Geometry: final body of the model. Coordinates: model frame, mm. A direction names the side the tool comes from. Coordinates: 2 decimals unless noted, no trailing zeros. Order: outer loops, then holes, each group sorted by start corner. A loop starts at its lowest first (then second) coordinate and runs counter-clockwise, first axis right, second up. Notation, with made-up numbers: (-21, 41) -> (-15, 41) arc R11 ccw to (-15, 45) -> close; hole circle Ø11 at (-16.75, 65.25). An arc over 180 degrees is marked (long way). Use CSV: the item, a comma, the result in double quotes. Start each with the question number.
from build123d import *

# Parameters (mm, degrees)
F0_R          = 35
F1_DEPTH      = 2
F2_R          = 29
F3_DEPTH      = 5
F4_R          = 27
F5_DEPTH      = 5
F6_W          = 45.179169625
F6_H          = 45.1430678368
F7_DEPTH      = 2.001
F7_DEPTH_BACK = 5.001
F8_R          = 4.99999
F9_R          = 10


# Not quite as in the source:
# - a fillet or chamfer is up to 0.001 mm smaller than in the source, because OpenCascade refuses the exact size


with BuildPart() as f1:
    # F0 (on Top) → F1 (new body)
    with BuildSketch(Plane.XY):
        Circle(F0_R)
    extrude(amount=F1_DEPTH)

    # F2 (on face) → F3 (join)
    with BuildSketch(Plane.XY.offset(2)):
        Circle(F2_R)
    extrude(amount=F3_DEPTH)

    # F4 (on face) → F5 (cut, through all)
    with BuildSketch(Plane.XY.offset(7)):
        Circle(F4_R)
    extrude(amount=-F5_DEPTH, mode=Mode.SUBTRACT)

    # F6 (on face) → F7 (cut, two sides)
    with BuildSketch(Plane.XY.offset(2)) as f7_sk:
        with Locations((-22.5895848125, 22.5715339184)):
            Rectangle(F6_W, F6_H)
    extrude(amount=-F7_DEPTH, mode=Mode.SUBTRACT)
    extrude(f7_sk.sketch, amount=F7_DEPTH_BACK, mode=Mode.SUBTRACT)

    # F8 (radius 5 in the source; OpenCascade refuses exactly that, so slightly less here)
    f8_edges = [f1.edges().sort_by_distance(p)[0] for p in [
        (19.091883, -19.091883, 2),
    ]]
    fillet(f8_edges, radius=F8_R)

    # F9
    f9_edges = [f1.edges().sort_by_distance(p)[0] for p in [
        (0, 0, 1),
    ]]
    fillet(f9_edges, radius=F9_R)


solid = f1.part
(1) Access query for faces 4 (the face through (-23, 0, 1)), 5 (the face through (20, -21, 4)), 6 (the face through (23.92, -25.55, 0.99)). Directions: +Z, -Z, +X, -X, +Y, -Y. A direction counts if a zero-diameter tool reaches every point of the face in a straight line with its end or side. Return the directions, or none.
(2) Line query: line 1 (Z direction, x = 9, y = -15); line 2 (X direction, y = 13.5, z = 5.75); line 3 (Y direction, x = -9, z = 6.5). Output: solid intervals per line, ascending. Write a range as from..to.
(3) Section B-B (x = 30.5). Return loops of the section in (y, z).
(4) Section A-A (z = 1). Return loops of the section in (x, y), then the cut area to 3 significant figures.
(5) First-contact query: pin 1 (4 mm diameter, centred on x = 8, z = 6, fed in from -Y); pin 2 (1 mm diameter, centred on x = -26.5, z = 3.5, fed in from +Y). Flat tips, straight axial feed; report the tip coordinate or a pass-through.
(6) Mould query, pull axis Y, two halves, no side actions, for faces 1 (the face through (-2.85, 3.01, 0.99)), 2 (the face through (7, -7, 0)), 3 (the face through (5, -5, 2)). Classes: pulls with the +Y half, pulls with the -Y half, needs draft (parallel to the pull), parting line crosses it, or undercut.
Check sheet entries:
1,face 4,"+Z, -Z, -X, +Y"
1,face 5,"+Z"
1,face 6,"+Z, -Z"
2,line 1,"z = 0..2"
2,line 2,"x = 23.2..25.67"
2,line 3,"y = -27.57..-25.43"
3,outline,"(-17.17, 0) -> (17.17, 0) -> (17.17, 2) -> (-17.17, 2) -> close"
4,outline,"(-35, 0) arc R35 ccw (long way) to (0, 35) -> (0, 10) arc R10 cw to (-10, 0) -> close"
4,area,"2,910 mm^2"
5,pin 1,"stops at y = -28.37"
5,pin 2,"stops at y = 0"
6,face 1,"pulls with the +Y half"
6,face 2,"needs draft"
6,face 3,"undercut"
